Answer from the drawing. Dimensions are ordinates in mm from the lowest x, y and z of the part. A direction names the side the tool comes from. Coordinates: 2 decimals unless noted, no trailing zeros. Write each loop counter-clockwise with the first axis right and the second up, starting at its lowest first coordinate (ties: lowest second). Pieces come first, ordered by that corner, then holes.
(1) Which of the six approach directions +Z, -Z, +X, -X, +Y, -Y give full straight-line access (tool end or side, diameter ignored) to the marked faces 4, 5 and 6?
(2) Given pin 1 (1 mm diameter, centred on y = 0.5, z = 3.5, fed in from -X); pin 2 (1.5 mm diameter, centred on y = 2.5, z = 8, fed in from -X), each flat-ended and moving along its own axis, determine where each tip first touches the part or whether it passes through.
(3) Find the intervals of material crossed by probe 1 along X at (y, z) = (2.35, 11.75); probe 2 along X at (y, z) = (1.5, 5.75); probe 3 along Z at (x, y) = (7.5, 1.1), in increasing order.
(4) Section C-C on x = 11 is taken. Write down the section's boundary in (y, z), then the cut area to 3 significant figures.
(5) The mould has two halves that part along X. Classify the marked faces 1, 2 and 3: +X half, -X half, draft (parallel to the pull), parting line (faces both ways), or undercut.
(6) Section A-A on z = 7.5 is taken. Write down the section's boundary in (x, y).
(7) Section D-D on x = 13.5 is taken. Write down the section's boundary in (y, z), then the cut area to 3 significant figures.
(8) Section B-B on y = 1.2 is taken. Write down the section's boundary in (x, z).
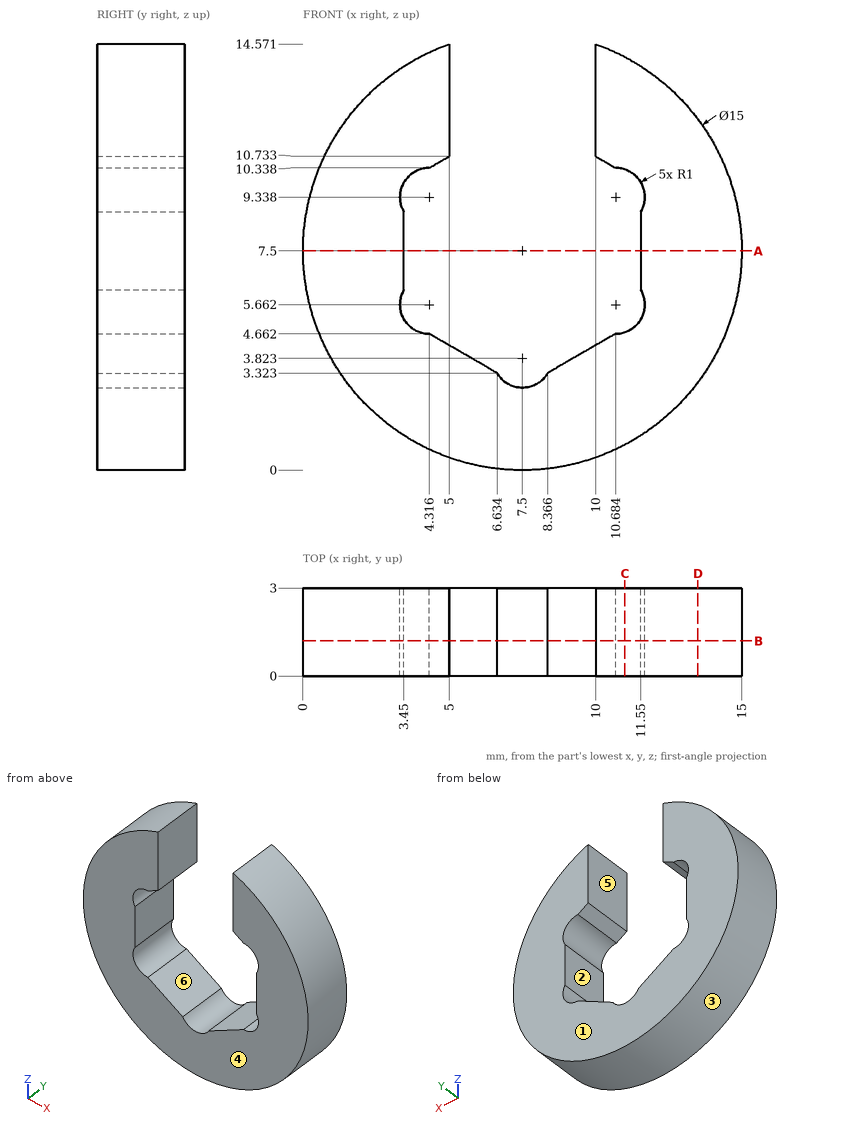
Response:
1. face 4: +Z, -Z, +X, -X, -Y
1. face 5: +Z, +Y, -Y
1. face 6: +Y, -Y
2. pin 1: stops at x = 0.87
2. pin 2: stops at x = 0
3. probe 1: x = 1.32 to 5, 10 to 13.68
3. probe 2: x = 0.21 to 3.32, 11.68 to 14.79
3. probe 3: z = 0 to 2.82
4. outline: (0, 0.87) - (3, 0.87) - (3, 4.71) - (0, 4.71) - close; (0, 10.29) - (3, 10.29) - (3, 14.13) - (0, 14.13) - close
4. area: 23.1 mm2
5. face 1: draft
5. face 2: undercut
5. face 3: parting line
6. outline: (0, 0) - (3.45, 0) - (3.45, 3) - (0, 3) - close; (11.55, 0) - (15, 0) - (15, 3) - (11.55, 3) - close
7. outline: (0, 3) - (3, 3) - (3, 12) - (0, 12) - close
7. area: 27.0 mm2
8. outline: (3.45, 6.16) - (3.45, 8.84) arc R1 cw to (4.32, 10.34) - (5, 10.73) - (5, 14.57) arc R7.5 ccw (long way) to (10, 14.57) - (10, 10.73) - (10.68, 10.34) arc R1 cw to (11.55, 8.84) - (11.55, 6.16) arc R1 cw to (10.68, 4.66) - (8.37, 3.32) arc R1 cw to (6.63, 3.32) - (4.32, 4.66) arc R1 cw to start
